from build123d import *

# Parameters (mm, degrees)
SKETCH1_W                = 34.29
SKETCH1_H                = 28.575
BOSS_EXTRUDE1_DEPTH      = 23
SKETCH3_R                = 12.446
CUT_EXTRUDE1_DEPTH       = 21
SKETCH5_R                = 1.625
SKETCH5_R_2              = 3.75
CUT_EXTRUDE2_DEPTH       = 3
SKETCH7_W                = 8.89
SKETCH7_H                = 12.7
BOSS_EXTRUDE2_DEPTH      = 3.81
BOSS_EXTRUDE2_DEPTH_BACK = 5.08


with BuildPart() as part:
    # Sketch1 → Boss-Extrude1 (new body)
    with BuildSketch(Plane.XY):
        Rectangle(SKETCH1_W, SKETCH1_H)
    extrude(amount=BOSS_EXTRUDE1_DEPTH)

    # Sketch3 → Cut-Extrude1 (cut)
    with BuildSketch(Plane.XY.offset(23)):
        Circle(SKETCH3_R)
    extrude(amount=-CUT_EXTRUDE1_DEPTH, mode=Mode.SUBTRACT)

    # Sketch5 → Cut-Extrude2 (cut, through all)
    with BuildSketch(Plane.XY.offset(2)):
        with Locations((0, 8.5)):
            Circle(SKETCH5_R)
        with Locations((-8.5, 0)):
            Circle(SKETCH5_R)
        with Locations((8.5, 0)):
            Circle(SKETCH5_R)
        with Locations((0, -8.5)):
            Circle(SKETCH5_R)
        Circle(SKETCH5_R_2)
    extrude(amount=-CUT_EXTRUDE2_DEPTH, mode=Mode.SUBTRACT)

    # Sketch7 → Boss-Extrude2 (add, two sides)
    with BuildSketch(Plane.XY.offset(23)) as boss_extrude2_sk:
        with Locations((-21.59, -7.9375)):
            Rectangle(SKETCH7_W, SKETCH7_H)
        with Locations((21.59, -7.9375)):
            Rectangle(SKETCH7_W, SKETCH7_H)
    extrude(amount=BOSS_EXTRUDE2_DEPTH)
    extrude(boss_extrude2_sk.sketch, amount=-BOSS_EXTRUDE2_DEPTH_BACK)


solid = part.part
Work out the finished part from the listing and answer in its coordinate system (mm). A direction names the side the tool comes from. Coordinates: 2 decimals unless noted, no trailing zeros. Write each loop counter-clockwise with the first axis right and the second up, starting at its lowest first coordinate (ties: lowest second). Pieces come first, ordered by that corner, then holes. Notation, with made-up numbers: M 74,-39 L 107,-39 A16 ccw 107,-23 Z; hole C 30.5,44 d11. An arc over 180 degrees is marked long. Write item = value, one per line.
1. For faces 5 (the face through (-8, 10, 23)), 6 (the face through (22, -1.588, 22)), 7 (the face through (-2.7, -12.15, 12.65)), determine the directions among +Z, -Z, +X, -X, +Y, -Y from which every point of the face is accessible in a straight line to the end or side of a thin tool.
Solution:
face_5 = +Z, +Y, -Y
face_6 = +Z, -Z, +X, +Y
face_7 = +Z
2. The part is cut by section D-D (z = 24.5). Determine the outline of the cut face in (x, y) (1 decimal), then the cut area to 3 significant figures.
Solution:
outline = M -26,-14.3 L -17.1,-14.3 L -17.1,-1.6 L -26,-1.6 Z; M 17.1,-14.3 L 26,-14.3 L 26,-1.6 L 17.1,-1.6 Z
area = 226 mm2
3. Straight lines are drawn through the part: line 1 (Z direction, x = 10, y = -2.75); line 2 (Y direction, x = -8.5, z = 1.25) (1 decimal); line 3 (Z direction, x = 12.5, y = -11.75). For each, find the intervals that lie inside material, in ascending order. Write a range as from..to.
Solution:
line_1 = 0..2
line_2 = -14.3..-1.6, 1.6..14.3
line_3 = 0..23
4. Flat-ended cylindrical pins translate along their axes: pin 1 (1.5 mm diameter, centred on y = 0.5, z = 12, fed in from +X) (3 decimals); pin 2 (7 mm diameter, centred on x = -21.5, z = 24, fed in from +Y); pin 3 (6 mm diameter, centred on x = 3.5, y = -2, fed in from +Z). Find the tip coordinate at first contact, or state that the pin passes through.
Solution:
pin_1 = 17.145
pin_2 = -1.59
pin_3 = 2
5. The part is cut by section C-C (z = 21.75). Determine the outline of the cut face in (x, y) (1 decimal).
Solution:
outline = M -26,-14.3 L 26,-14.3 L 26,-1.6 L 17.1,-1.6 L 17.1,14.3 L -17.1,14.3 L -17.1,-1.6 L -26,-1.6 Z; hole C 0,0 d24.9
6. The part is cut by section A-A (y = 0). Determine the outline of the cut face in (x, z) (3 decimals), then the cut area to 3 significant figures.
Solution:
outline = M -17.145,0 L -10.125,0 L -10.125,2 L -12.446,2 L -12.446,23 L -17.145,23 Z; M -6.875,0 L -3.75,0 L -3.75,2 L -6.875,2 Z; M 3.75,0 L 6.875,0 L 6.875,2 L 3.75,2 Z; M 10.125,0 L 17.145,0 L 17.145,23 L 12.446,23 L 12.446,2 L 10.125,2 Z
area = 238 mm2
7. Determine the mould class of faces 1 (the face through (-22, -1.588, 22)), 2 (the face through (3, 3, 2)), 3 (the face through (17.145, -8, 25)), 4 (the face through (-3.746, 0.165, 1.014)) for opening direction Y: released by +Y, released by -Y, zero draft, split by the parting line, or undercut.
Solution:
face_1 = released by +Y
face_2 = undercut
face_3 = zero draft
face_4 = undercut
8. The part is cut by section B-B (x = 0). State how many separate pieces and enclosed holes the cut face has, then the cut area to 3 significant figures.
Solution:
separate_pieces = 4
enclosed_holes = 0
area = 106 mm2
